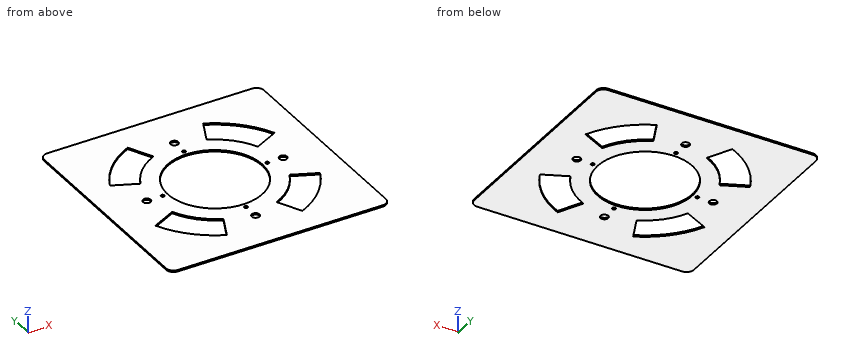
```python
from build123d import *

# Parameters (mm, degrees)
F0_R     = 2.25
F0_R_2   = 62.5
F1_DEPTH = 2
F2_R     = 5.1
F3_DEPTH = 25
F5_DEPTH = 25


with BuildPart() as f1:
    # F0 (on Top) → F1 (new body)
    with BuildSketch(Plane.XY):
        with BuildLine():
            Line((135, 145), (-135, 145))
            ThreePointArc((-135, 145), (-142.071068, 142.071068), (-145, 135))
            Line((-145, 135), (-145, -135))
            ThreePointArc((-145, -135), (-142.071068, -142.071068), (-135, -145))
            Line((-135, -145), (135, -145))
            ThreePointArc((135, -145), (142.071068, -142.071068), (145, -135))
            Line((145, -135), (145, 135))
            ThreePointArc((145, 135), (142.071068, 142.071068), (135, 145))
        make_face()
        with Locations((0, -69)):
            Circle(F0_R, mode=Mode.SUBTRACT)
        with Locations((-69, 0)):
            Circle(F0_R, mode=Mode.SUBTRACT)
        Circle(F0_R_2, mode=Mode.SUBTRACT)
        with Locations((69, 0)):
            Circle(F0_R, mode=Mode.SUBTRACT)
        with Locations((0, 69)):
            Circle(F0_R, mode=Mode.SUBTRACT)
    extrude(amount=F1_DEPTH)

    # F2 (on face) → F3 (cut)
    with BuildSketch(Plane.XY.offset(2)):
        with Locations((0, 90)):
            Circle(F2_R)
        with Locations((-90, 0)):
            Circle(F2_R)
        with Locations((0, -90)):
            Circle(F2_R)
        with Locations((90, 0)):
            Circle(F2_R)
    extrude(amount=-F3_DEPTH, mode=Mode.SUBTRACT)

    # F4 (on face) → F5 (cut)
    with BuildSketch(Plane.XY.offset(2)):
        with BuildLine():
            Line((-35, 77.459667), (-50.635936, 108.772883))
            ThreePointArc((-50.635936, 108.772883), (-85.317456, 84.359171), (-109.337881, 49.404109))
            Line((-109.337881, 49.404109), (-77.459667, 35))
            ThreePointArc((-77.459667, 35), (-60.104076, 60.104076), (-35, 77.459667))
        make_face()
        with BuildLine():
            Line((77.459667, 35), (108.772883, 50.635936))
            ThreePointArc((108.772883, 50.635936), (84.359171, 85.317456), (49.404109, 109.337881))
            Line((49.404109, 109.337881), (35, 77.459667))
            ThreePointArc((35, 77.459667), (60.104076, 60.104076), (77.459667, 35))
        make_face()
        with BuildLine():
            ThreePointArc((50.635936, -108.772883), (85.317456, -84.359171), (109.337881, -49.404109))
            Line((109.337881, -49.404109), (77.459667, -35))
            ThreePointArc((77.459667, -35), (60.104076, -60.104076), (35, -77.459667))
            Line((35, -77.459667), (50.635936, -108.772883))
        make_face()
        with BuildLine():
            ThreePointArc((-108.772883, -50.635936), (-84.359171, -85.317456), (-49.404109, -109.337881))
            Line((-49.404109, -109.337881), (-35, -77.459667))
            ThreePointArc((-35, -77.459667), (-60.104076, -60.104076), (-77.459667, -35))
            Line((-77.459667, -35), (-108.772883, -50.635936))
        make_face()
    extrude(amount=-F5_DEPTH, mode=Mode.SUBTRACT)


solid = f1.part
```
Input: part model. Units: mm. Frame: model coordinates. Round coordinates to 2 decimals unless told otherwise and drop trailing zeros. Loops run counter-clockwise (first coordinate to the right, second up) from the corner with the lowest first, then second, coordinate; pieces in that order, holes last. Notation, with made-up numbers: (19.5, 89.5) -> (67.5, 89.5) arc R18 ccw to (67.5, 119.5) -> close; hole circle Ø5 at (44.5, 40). An arc over 180 degrees is marked (long way). Write each question's results on one line, items separated by ' | '.
1. Section A-A (z = 1.3). State how many separate pieces and enclosed holes the cut face has, and give its area (3 significant figures).
Geometry results:
separate pieces: 1 | enclosed holes: 13 | area: 61,100 mm2
2. Section D-D (y = -90). Return loops of the section in (x, z), and give its area (3 significant figures).
Geometry results:
outline: (-145, 0) -> (-79.34, 0) -> (-79.34, 2) -> (-145, 2) -> close; (-40.67, 0) -> (-5.1, 0) -> (-5.1, 2) -> (-40.67, 2) -> close; (5.1, 0) -> (41.26, 0) -> (41.26, 2) -> (5.1, 2) -> close; (79.34, 0) -> (145, 0) -> (145, 2) -> (79.34, 2) -> close | area: 406 mm2
3. Section C-C (y = -13). Return loops of the section in (x, z).
Geometry results:
outline: (-145, 0) -> (-61.13, 0) -> (-61.13, 2) -> (-145, 2) -> close; (61.13, 0) -> (145, 0) -> (145, 2) -> (61.13, 2) -> close
4. Ray query, line 1 (Y direction, x = 0, z = 1.6); line 2 (X direction, y = -38, z = 1.25); line 3 (X direction, y = -75, z = 0.35). Return the intervals inside material, ascending. Write a range as from..to.
Geometry results:
line 1: -145..-95.1, -84.9..-71.25, -66.75..-62.5, 62.5..66.75, 71.25..84.9, 95.1..145 | line 2: -145..-83.47, -76.03..-49.62, 49.62..76.03, 84.1..145 | line 3: -145..-93.65, -40..40, 93.65..145
5. Section B-B (x = 22). Return loops of the section in (y, z), and give its area (3 significant figures).
Geometry results:
outline: (-145, 0) -> (-58.5, 0) -> (-58.5, 2) -> (-145, 2) -> close; (58.5, 0) -> (145, 0) -> (145, 2) -> (58.5, 2) -> close | area: 346 mm2
